Autodesk Inventor part; units mm, degrees
ref_plane "YZ Plane" through (0, 0, 0) normal (1, 0, 0) x (0, 1, 0)
ref_plane "XZ Plane" through (0, 0, 0) normal (0, 1, 0) x (-1, 0, 0)
ref_plane "XY Plane" through (0, 0, 0) normal (0, 0, 1) x (1, 0, 0)
sketch "Sketch1" plane through (0, 0, 0) normal (0, 0, 1) x (1, 0, 0)
  line L0 (-15, -28.975) -> (-15, -0.175)
  arc A0 (-15, -28.975) -> (-13, -30.975) centre (-13, -28.975) ccw
  line L1 (13, -30.975) -> (-13, -30.975)
  arc A1 (13, -30.975) -> (15, -28.975) centre (13, -28.975) ccw
  line L2 (15, -0.175) -> (15, -28.975)
  line L3 (45, -0.175) -> (15, -0.175)
  line L4 (45, 62.125) -> (45, -0.175)
  line L5 (-15, -0.175) -> (-45, -0.175)
  circle A2 centre (7.5, -27.775) radius 1.75
  circle A3 centre (7.5, -9.775) radius 1.75
  circle A4 centre (-7.5, -9.775) radius 1.75
  circle A5 centre (-7.5, -27.775) radius 1.75
  line L6 (-45, 62.125) -> (45, 62.125)
  line L7 (-45, -0.175) -> (-45, 62.125)
  point P0 (0, 0)
  point P1 (-45, 30.975)
extrude "Extrusion1" add sketch "Sketch1" along normal blind 1.5
sketch "Sketch2" plane through (0, 0, 1.5) normal (0, 0, 1) x (1, 0, 0)
  line L0 (-45, 30.975) -> (45, 30.975)
  line L1 (45, 62.125) -> (45, 30.975)
  line L2 (-45, 62.125) -> (45, 62.125)
  line L3 (-45, 30.975) -> (-45, 62.125)
  line L4 (15, -28.975) -> (15, -0.175)
  line L5 (15, -0.175) -> (45, -0.175)
  line L6 (45, -0.175) -> (45, 62.125)
  line L7 (-45, -0.175) -> (-15, -0.175)
  line L8 (-15, -0.175) -> (-15, -28.975)
  arc A0 (-15, -28.975) -> (-13, -30.975) centre (-13, -28.975) ccw
  line L9 (-13, -30.975) -> (13, -30.975)
  arc A1 (13, -30.975) -> (15, -28.975) centre (13, -28.975) ccw
  circle A2 centre (7.5, -27.775) radius 1.75
  circle A3 centre (7.5, -9.775) radius 1.75
  circle A4 centre (-7.5, -9.775) radius 1.75
  circle A5 centre (-7.5, -27.775) radius 1.75
  line L10 (45, 62.125) -> (-45, 62.125)
  line L11 (-45, 62.125) -> (-45, -0.175)
  point P0 (0, 0)
extrude "Extrusion2" add sketch "Sketch2" along normal blind 1.5
sketch "Sketch3" plane through (0, 0, 3) normal (0, 0, 1) x (1, 0, 0)
  line L0 (45, 62.125) -> (-45, 62.125)
  line L1 (-45, 62.125) -> (-45, -0.175)
  line L2 (-45, -0.175) -> (-15, -0.175)
  line L3 (-15, -0.175) -> (-15, -28.975)
  arc A0 (-15, -28.975) -> (-13, -30.975) centre (-13, -28.975) ccw
  line L4 (-13, -30.975) -> (13, -30.975)
  arc A1 (13, -30.975) -> (15, -28.975) centre (13, -28.975) ccw
  line L5 (15, -28.975) -> (15, -0.175)
  line L6 (15, -0.175) -> (45, -0.175)
  line L7 (45, -0.175) -> (45, 62.125)
  circle A2 centre (7.5, -27.775) radius 1.75
  circle A3 centre (7.5, -9.775) radius 1.75
  circle A4 centre (-7.5, -9.775) radius 1.75
  circle A5 centre (-7.5, -27.775) radius 1.75
  circle A6 centre (0, -18.775) radius 2.6186
  line L8 (-13, -30.975) -> (13, -30.975)
  line L9 (0, -13.8344) -> (4.5, -13.8344)
  line L10 (4.5, -13.8344) -> (4.5, -30.975)
  line L11 (4.5, -30.975) -> (0, -30.975)
  line L12 (0, -30.975) -> (0, -13.8344)
  line L13 (0, -13.8344) -> (-4.5, -13.8344)
  line L14 (-4.5, -13.8344) -> (-4.5, -30.975)
  point P0 (0, 0)
  dimension "d4" = 4.5
extrude "Extrusion3" cut sketch "Sketch3" against normal through all contours L4 L12 A6 L9 L10 | L14 L13 L12 A6 L4 | L12 A6 | A6 L12
sketch "Sketch4" plane through (0, 0, 1.5) normal (0, 0, -1) x (-1, 0, 0)
  circle A0 centre (7.5, -27.775) radius 1.75
  circle A1 centre (7.5, -9.775) radius 1.75
  circle A2 centre (-7.5, -9.775) radius 1.75
  circle A3 centre (-7.5, -27.775) radius 1.75
  line L0 (4.5, -30.975) -> (4.5, -13.8344)
  line L1 (4.5, -13.8344) -> (-4.5, -13.8344)
  line L2 (-4.5, -13.8344) -> (-4.5, -30.975)
  line L3 (-4.5, -30.975) -> (-13, -30.975)
  arc A4 (-15, -28.975) -> (-13, -30.975) centre (-13, -28.975) ccw
  line L4 (-15, -28.975) -> (-15, -0.175)
  line L5 (-15, -0.175) -> (-45, -0.175)
  line L6 (-45, -0.175) -> (-45, 62.125)
  line L7 (-45, 62.125) -> (45, 62.125)
  line L8 (45, 62.125) -> (45, -0.175)
  line L9 (45, -0.175) -> (15, -0.175)
  line L10 (15, -0.175) -> (15, -28.975)
  arc A5 (13, -30.975) -> (15, -28.975) centre (13, -28.975) ccw
  line L11 (13, -30.975) -> (4.5, -30.975)
  line L12 (-45, 30.975) -> (45, 30.975)
  point P0 (0, 0)
extrude "Extrusion4" [suppressed]
properties part number "lead_1" material "Lead"
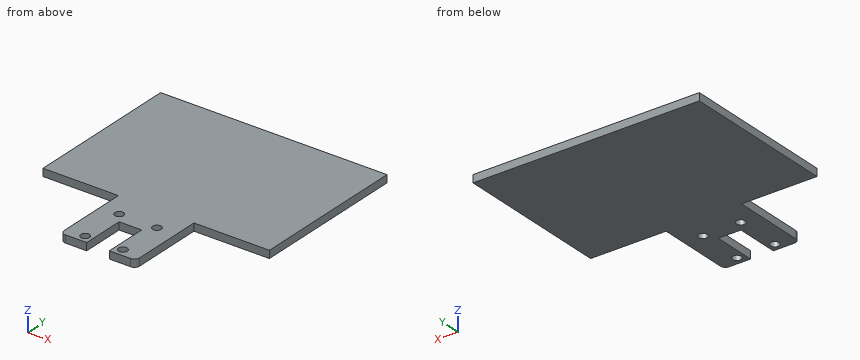
Check sheet for the modelled part. Datum: model origin and axes. Units: mm. Round coordinates to 2 decimals unless told otherwise and drop trailing zeros. Loops run counter-clockwise (first coordinate to the right, second up) from the corner with the lowest first, then second, coordinate; pieces in that order, holes last.
1. Sectioned sample at A-A on y = -24. Record the boundary of the cut face in (x, z).
2. Scan lines: probe 1 along Y at (x, z) = (-7.5, 2) (3 decimals); probe 2 along X at (y, z) = (-27, 2.8); probe 3 along X at (y, z) = (-4, 1.1). Record each from-to range of solid material in increasing order.
3. Gauge pin test, flat ends, axial feed: pin 1 Ø3 at (x, y) = (-7.5, -9.775) entering from +Z; pin 2 Ø1.5 at (x, z) = (-3.5, 2) entering from -Y; pin 3 Ø1.5 at (y, z) = (-13.5, 2) entering from -X; pin 4 Ø1.5 at (x, z) = (-31, 1) entering from -Y (3 decimals). Record the tip position at first contact, or that the pin passes through.
4. Sectioned sample at C-C on z = 1.4. Record the boundary of the cut face in (x, y) (3 decimals), and give its area (3 significant figures).
5. Sectioned sample at D-D on x = 28. Record the boundary of the cut face in (y, z) (3 decimals), and give its area (3 significant figures).
6. Sectioned sample at B-B on x = -7.5. Record the boundary of the cut face in (y, z) (3 decimals).
Recorded:
1. outline: (-15, 0) - (-4.5, 0) - (-4.5, 3) - (-15, 3) - close; (4.5, 0) - (15, 0) - (15, 3) - (4.5, 3) - close
2. probe 1: y = -30.975 to -29.525, -26.025 to -11.525, -8.025 to 62.125
2. probe 2: x = -15 to -9.07, -5.93 to -4.5, 4.5 to 5.93, 9.07 to 15
2. probe 3: x = -15 to 15
3. pin 1: passes through
3. pin 2: stops at y = -13.83
3. pin 3: stops at x = -15
3. pin 4: stops at y = -0.175
4. outline: (-45, -0.175) - (-15, -0.175) - (-15, -28.975) arc R2 ccw to (-13, -30.975) - (-4.5, -30.975) - (-4.5, -13.834) - (4.5, -13.834) - (4.5, -30.975) - (13, -30.975) arc R2 ccw to (15, -28.975) - (15, -0.175) - (45, -0.175) - (45, 62.125) - (-45, 62.125) - close; hole circle Ø3.5 at (-7.5, -27.775); hole circle Ø3.5 at (-7.5, -9.775); hole circle Ø3.5 at (7.5, -27.775); hole circle Ø3.5 at (7.5, -9.775)
4. area: 6,340 mm2
5. outline: (-0.175, 0) - (62.125, 0) - (62.125, 3) - (-0.175, 3) - close
5. area: 187 mm2
6. outline: (-30.975, 0) - (-29.525, 0) - (-29.525, 3) - (-30.975, 3) - close; (-26.025, 0) - (-11.525, 0) - (-11.525, 3) - (-26.025, 3) - close; (-8.025, 0) - (62.125, 0) - (62.125, 3) - (-8.025, 3) - close
